from build123d import *

# Parameters (mm, degrees)
F0_W     = 54
F0_H     = 82
F0_R     = 2.5
F0_R_2   = 8
F1_DEPTH = 5
F2_R     = 1


with BuildPart() as f1:
    # F0 (on Top) → F1 (new body)
    with BuildSketch(Plane.XY):
        Rectangle(F0_W, F0_H)
        with Locations((-19, -33)):
            Circle(F0_R, mode=Mode.SUBTRACT)
        with Locations((0, -26)):
            Circle(F0_R_2, mode=Mode.SUBTRACT)
        with Locations((19, -33)):
            Circle(F0_R, mode=Mode.SUBTRACT)
        with Locations((-19, 0)):
            Circle(F0_R, mode=Mode.SUBTRACT)
        with Locations((-19, 33)):
            Circle(F0_R, mode=Mode.SUBTRACT)
        with Locations((19, 0)):
            Circle(F0_R, mode=Mode.SUBTRACT)
        with Locations((0, 26)):
            Circle(F0_R_2, mode=Mode.SUBTRACT)
        with Locations((19, 33)):
            Circle(F0_R, mode=Mode.SUBTRACT)
    extrude(amount=F1_DEPTH)

    # F2
    f2_edges = [f1.edges().sort_by_distance(p)[0] for p in [
        (27, -41, 2.5),
        (-27, -41, 2.5),
        (-27, 41, 2.5),
        (27, 41, 2.5),
    ]]
    fillet(f2_edges, radius=F2_R)


solid = f1.part
For this review, take the finished solid that the model builds, in its own axes (mm). Give positions to 0.01 mm unless a question says otherwise; leave off trailing zeros. Order: outer loops, then holes, each group sorted by start corner. A loop starts at its lowest first (then second) coordinate and runs counter-clockwise, first axis right, second up. Notation, with made-up numbers: M 87.5,46 L 106.5,46 A31 cw 106.5,82 Z; hole C -24.75,-27 d1. An arc over 180 degrees is marked long. Answer in a Markdown table with one row per item. Add a question column.
(1) Consider section D-D on z = 2.55. Give the number of separate pieces and of enclosed holes in the cut face, and give its area (3 significant figures).
(2) For pin 1 (8 mm diameter, centred on x = -19, y = 0, fed in from +Z), flat-tipped, find the tip position at first contact; note if it passes through.
(3) Wall thickness on probe 1 along Y at (x, z) = (0.5, 1); probe 2 along Y at (x, z) = (-19, 3.25); probe 3 along X at (y, z) = (34.5, 2.1): over which ranges is each line inside the solid? List them lowest first. Write a range as [from, to].
(4) Consider section A-A on x = 0. State the section outline as (y, z) points, and give its area (3 significant figures).
(5) Consider section C-C on x = 19. State the section outline as (y, z) points.
(6) Mouldability with a two-part tool opening along X and no side actions: class faces 1 (the face through (0, 1, 0)), 2 (the face through (-27, -1, 2)), 3 (the face through (-1.73, -33.81, 2.46)) as +X half, -X half, draft (parallel to the pull), parting line (faces both ways), or undercut.
(7) Consider section B-B on y = 26. State the section outline as (x, z) points.
Evaluation:
| question | item | result |
|---|---|---|
| 1 | separate pieces | 1 |
| 1 | enclosed holes | 8 |
| 1 | area | 3,910 mm^2 |
| 2 | pin 1 | stops at z = 5 |
| 3 | probe 1 | y = [-41, -33.98], [-18.02, 18.02], [33.98, 41] |
| 3 | probe 2 | y = [-41, -35.5], [-30.5, -2.5], [2.5, 30.5], [35.5, 41] |
| 3 | probe 3 | x = [-27, -21], [-17, 17], [21, 27] |
| 4 | outline | M -41,0 L -34,0 L -34,5 L -41,5 Z; M -18,0 L 18,0 L 18,5 L -18,5 Z; M 34,0 L 41,0 L 41,5 L 34,5 Z |
| 4 | area | 250 mm^2 |
| 5 | outline | M -41,0 L -35.5,0 L -35.5,5 L -41,5 Z; M -30.5,0 L -2.5,0 L -2.5,5 L -30.5,5 Z; M 2.5,0 L 30.5,0 L 30.5,5 L 2.5,5 Z; M 35.5,0 L 41,0 L 41,5 L 35.5,5 Z |
| 6 | face 1 | draft |
| 6 | face 2 | -X half |
| 6 | face 3 | undercut |
| 7 | outline | M -27,0 L -8,0 L -8,5 L -27,5 Z; M 8,0 L 27,0 L 27,5 L 8,5 Z |
